Part model, mm, in its own coordinate system. Give positions to 0.01 mm unless a question says otherwise; leave off trailing zeros. Order: outer loops, then holes, each group sorted by start corner. A loop starts at its lowest first (then second) coordinate and runs counter-clockwise, first axis right, second up. Notation, with made-up numbers: (19, 25) -> (51, 25) arc R21 cw to (51, 38) -> close; hole circle Ø2 at (9, 33.5). An arc over 180 degrees is marked (long way). Write item = value, one per line. Start each with the question number.
(1) Saw through at C-C, the plane y = -8. List the corners of the cut face in (x, z).
(2) Flat gauge pins, fed straight in: pin 1 (8 mm diameter, centred on x = 36.22, y = -9.71, fed in from -Z); pin 2 (3 mm diameter, centred on y = -18.5, z = 4.5, fed in from -X); pin 3 (1 mm diameter, centred on y = -14.5, z = 4, fed in from +X); pin 4 (1.5 mm diameter, centred on y = -42, z = 2.5, fed in from +X). Where does each tip first touch, or does it go through?
(3) Two-plate mould, pull along Y, no slides. Class faces 1 (the cylindrical face through (-30.48, -23.47, 2.47)), 2 (the cylindrical face through (-59.94, 2.64, 2.46)), 3 (the flat face through (-1, 1, 0)), 4 (the cylindrical face through (30.48, 23.47, 2.47)): pulls with the +Y half, pulls with the -Y half, needs draft (parallel to the pull), parting line crosses it, or undercut.
(4) Saw through at A-A, the plane x = 36. List the corners of the cut face in (y, z), then the cut area to 3 significant figures.
(5) Probe line 1 along Y through (x, z) = (32, 3.5); line 2 along X through (y, z) = (-29, 1.55); line 3 along Y through (x, z) = (-14, 3.55). List the from-to ranges inside material, lowest first. Write a range as from..to.
(6) Saw through at D-D, the plane x = 48. List the corners of the cut face in (y, z), then the cut area to 3 significant figures.
(7) Saw through at B-B, the plane z = 2.95. List the corners of the cut face in (x, y), then the cut area to 3 significant figures.
from build123d import *

# Parameters (mm, degrees)
F0_R            = 60
F1_DEPTH        = 5
F3_D            = 10
F3_COPIES_COUNT = 6


# Not quite as in the source:
# - a pattern or mirror of a feature is missing from the dataset's text; its kind, count and spacing are read off the source's solid


with BuildPart() as f1:
    # F0 (on Top) → F1 (new body)
    with BuildSketch(Plane.XY):
        Circle(F0_R)
    extrude(amount=F1_DEPTH)

    # F3 (through all)
    with Locations(Plane.XY.offset(5)):
        with Locations((26.5165042945, 26.5165042945)):
            f3 = Hole(F3_D / 2)

    # F3_copies: F3 ×6 about axis
    f3_copies_axis = Axis((0, 0, 0), (0, 0, 1))
    for i in range(1, F3_COPIES_COUNT):
        add(f3.rotate(f3_copies_axis, i * 360 / F3_COPIES_COUNT), mode=Mode.SUBTRACT)


solid = f1.part
Results list:
q1.outline = (-59.46, 0) -> (31.52, 0) -> (31.52, 5) -> (-59.46, 5) -> close; (40.92, 0) -> (59.46, 0) -> (59.46, 5) -> (40.92, 5) -> close
q2.pin_1 = through
q2.pin_2 = -57.54
q2.pin_3 = 58.34
q2.pin_4 = 43.57
q3.face_1 = undercut
q3.face_2 = parting line crosses it
q3.face_3 = needs draft
q3.face_4 = undercut
q4.outline = (-48, 0) -> (-14.7, 0) -> (-14.7, 5) -> (-48, 5) -> close; (-4.71, 0) -> (48, 0) -> (48, 5) -> (-4.71, 5) -> close
q4.area = 430 mm^2
q5.line_1 = -50.75..-12.38, -7.03..50.75
q5.line_2 = -52.53..-30.86, -22.18..52.53
q5.line_3 = -58.34..33.66, 38.78..58.34
q6.outline = (-36, 0) -> (36, 0) -> (36, 5) -> (-36, 5) -> close
q6.area = 360 mm^2
q7.outline = circle Ø120 at (0, 0); hole circle Ø10 at (-36.22, 9.71); hole circle Ø10 at (-26.52, -26.52); hole circle Ø10 at (-9.71, 36.22); hole circle Ø10 at (9.71, -36.22); hole circle Ø10 at (26.52, 26.52); hole circle Ø10 at (36.22, -9.71)
q7.area = 10,800 mm^2
